from build123d import *

# Parameters (mm, degrees)
F0_W     = 457.2
F0_H     = 609.6
F1_DEPTH = 876.3
F2_W     = 457.2
F2_H     = 101.6
F3_DEPTH = 101.6
F4_W     = 457.2
F4_H     = 774.7
F4_W_2   = 431.8
F4_H_2   = 279.4
F4_H_3   = 152.4
F5_DEPTH = 15.875


with BuildPart() as f1:
    # F0 (on Top) → F1 (new body)
    with BuildSketch(Plane.XY):
        with Locations((228.6, 304.8)):
            Rectangle(F0_W, F0_H)
    extrude(amount=F1_DEPTH)

    # F2 (on face) → F3 (cut)
    with BuildSketch(Plane.XZ):
        with Locations((228.6, 50.8)):
            Rectangle(F2_W, F2_H)
    extrude(amount=-F3_DEPTH, mode=Mode.SUBTRACT)

    # F4 (on face) → F5 (cut)
    with BuildSketch(Plane.XZ):
        with Locations((228.6, 488.95)):
            Rectangle(F4_W, F4_H)
        with Locations((228.6, 254)):
            Rectangle(F4_W_2, F4_H_2, mode=Mode.SUBTRACT)
        with Locations((228.6, 546.1)):
            Rectangle(F4_W_2, F4_H_2, mode=Mode.SUBTRACT)
        with Locations((228.6, 774.7)):
            Rectangle(F4_W_2, F4_H_3, mode=Mode.SUBTRACT)
    extrude(amount=-F5_DEPTH, mode=Mode.SUBTRACT)


solid = f1.part
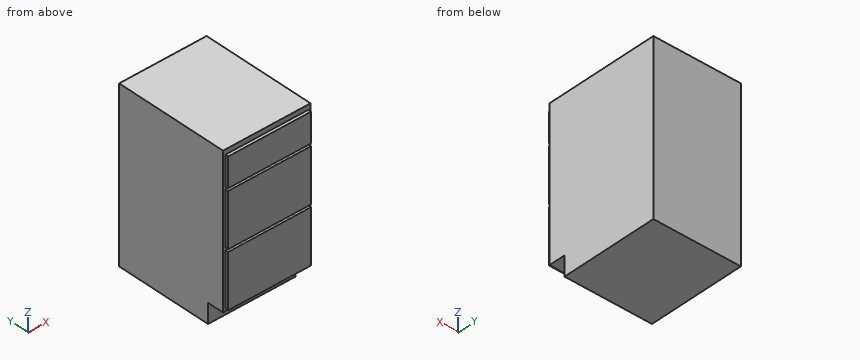
Here's how the part is built. I have some questions about the finished solid (model axes, mm). Coordinates: 2 decimals unless noted, no trailing zeros. Loops run counter-clockwise (first coordinate to the right, second up) from the corner with the lowest first, then second, coordinate; pieces in that order, holes last.
1. Imagine slicing it at A-A, the plane x = 364.5. Please give me the cut outline in (y, z) (3 decimals).
2. For P1, Ø5, axis at y = 6, z = 562, coming from the +X side; P2, Ø17.5, axis at x = 320, y = 5.5, coming from the -Z side; P3, Ø5, axis at y = 4.5, z = 228, coming from the -X side, each with a flat end and sliding along its axis, tell me the tip position at first contact or that it passes through.
3. I need wall thicknesses on L1, parallel to Y at x = 94, z = 398 (3 decimals); L2, parallel to Z at x = 415.5, y = 72; L3, parallel to Y at x = 215, z = 79. Which ranges of each line are inside material? Lowest first, please.
Taken from the geometry:
1. outline: (0, 114.3) - (15.875, 114.3) - (15.875, 101.6) - (101.6, 101.6) - (101.6, 0) - (609.6, 0) - (609.6, 876.3) - (15.875, 876.3) - (15.875, 850.9) - (0, 850.9) - (0, 698.5) - (15.875, 698.5) - (15.875, 685.8) - (0, 685.8) - (0, 406.4) - (15.875, 406.4) - (15.875, 393.7) - (0, 393.7) - close
2. P1: stops at x = 444.5
2. P2: stops at z = 114.3
2. P3: stops at x = 12.7
3. L1: y = 15.875 to 609.6
3. L2: z = 101.6 to 876.3
3. L3: y = 101.6 to 609.6
